For this review, use the dimensioned drawing (mm, ordinates from the lowest corner) and the shaded views. Round coordinates to 2 decimals unless told otherwise and drop trailing zeros. Write each loop counter-clockwise with the first axis right and the second up, starting at its lowest first coordinate (ties: lowest second). Pieces come first, ordered by that corner, then holes. Notation, with made-up numbers: M -12,-39 L 30,-39 A23 cw 30,-6 Z; hole C 27,-32.75 d11. An arc over 180 degrees is marked long. Use CSV: the item, a comma, the result in double quotes.
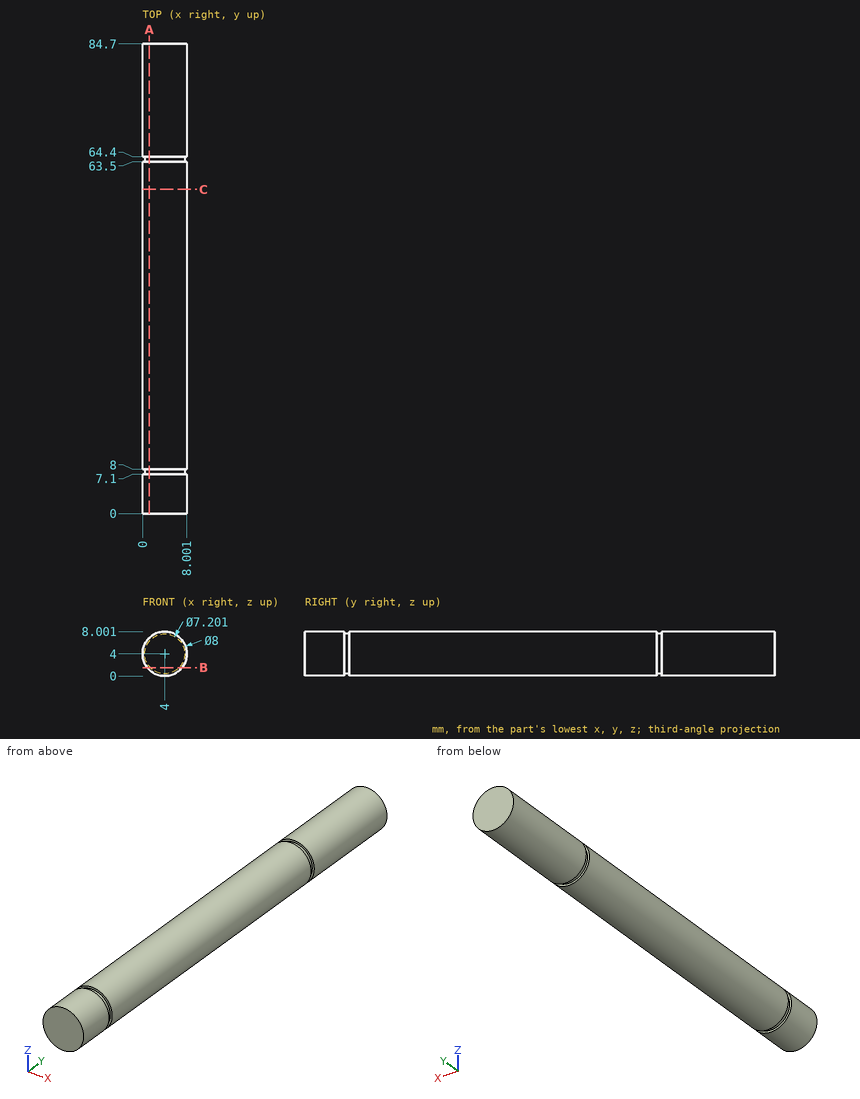
1) For pin 1 Ø3 at (x, y) = (2, 24.5) entering from -Z, flat-tipped, find the tip position at first contact; note if it passes through.
Answers:
pin 1,"z = 0.03"
2) Add section A-A on x = 1.25. Write out the cut boundary in (y, z) (1 decimal).
Answers:
outline,"M 0,1.1 L 7.1,1.1 L 7.1,1.7 L 8,1.7 L 8,1.1 L 63.5,1.1 L 63.5,1.7 L 64.4,1.7 L 64.4,1.1 L 84.7,1.1 L 84.7,6.9 L 64.4,6.9 L 64.4,6.3 L 63.5,6.3 L 63.5,6.9 L 8,6.9 L 8,6.3 L 7.1,6.3 L 7.1,6.9 L 0,6.9 Z"
3) Add section C-C on y = 58.5. Write out the cut boundary in (x, z).
Answers:
outline,"C 4,4 d8"
4) Add section B-B on z = 1.5. Write out the cut boundary in (x, y), then the cut area to 3 significant figures.
Answers:
outline,"M 0.88,0 L 7.12,0 L 7.12,7.1 L 6.59,7.1 L 6.59,8 L 7.12,8 L 7.12,63.5 L 6.59,63.5 L 6.59,64.4 L 7.12,64.4 L 7.12,84.7 L 0.88,84.7 L 0.88,64.4 L 1.41,64.4 L 1.41,63.5 L 0.88,63.5 L 0.88,8 L 1.41,8 L 1.41,7.1 L 0.88,7.1 Z"
area,"527 mm²"
5) Wall thickness on line 1 along Y through (x, z) = (1, 6.5); line 2 along Z through (x, y) = (3.75, 49.5): over which ranges is each line inside the solid? List them lowest first. Write a range as [from, to].
Answers:
line 1,"[0, 7.1], [8, 63.5], [64.4, 84.7]"
line 2,"[0.01, 7.99]"
